Model file for the job. Use its own axes, mm. A direction names the side the tool comes from. Round coordinates to 2 decimals unless told otherwise and drop trailing zeros. Order: outer loops, then holes, each group sorted by start corner. A loop starts at its lowest first (then second) coordinate and runs counter-clockwise, first axis right, second up. Notation, with made-up numbers: (26.25, 17) - (35.25, 17) arc R16 ccw to (35.25, 39) - close; hole circle Ø2 at (28, 34.5). An arc over 180 degrees is marked (long way). Write item = value, one per line.
```python
from build123d import *

# Parameters (mm, degrees)
F0_R     = 127
F1_DEPTH = 25.4
F3_DEPTH = 28.575
F5_DEPTH = 28.575


with BuildPart() as f1:
    # F0 (on Top) → F1 (new body)
    with BuildSketch(Plane.XY):
        Circle(F0_R)
    extrude(amount=F1_DEPTH)

    # F2 (on Right) → F3 (join, symmetric)
    with BuildSketch(Plane.YZ):
        Polygon((-107.95, 42.457951), (-107.95, 25.4), (0, 25.4), (0, 114.3), (-36.107951, 114.3), align=None)
        Polygon((0, 114.3), (0, 25.4), (107.95, 25.4), (107.95, 42.457951), (36.107951, 114.3), align=None)
    extrude(amount=F3_DEPTH, both=True)

    # F4 (on Front) → F5 (join, symmetric)
    with BuildSketch(Plane.XZ):
        Polygon((-114.3, 42.457951), (-114.3, 25.4), (0, 25.4), (0, 114.3), (-42.457951, 114.3), align=None)
        Polygon((0, 114.3), (0, 25.4), (114.3, 25.4), (114.3, 42.457951), (42.457951, 114.3), align=None)
    extrude(amount=F5_DEPTH, both=True)


solid = f1.part
```
1) 3-axis set-ups, long thin cutter, end or side, ignore diameter. For faces 1 (the face through (0, 107.95, 34)), 2 (the face through (0, -107.95, 34)), 3 (the face through (-63, 28.575, 61)), 4 (the face through (-63, -28.575, 61)), 5 (the face through (61, 28.575, 61)): which of +Z, -Z, +X, -X, +Y, -Y reach the whole face in a straight line?
Conclusion:
face_1 = +Z, +X, -X, +Y
face_2 = +Z, +X, -X, -Y
face_3 = +Z, -X, +Y
face_4 = +Z, -X, -Y
face_5 = +Z, +X, +Y
2) Cut at A-A (z = 34). Write the cut outline in (x, y) (3 decimals).
Conclusion:
outline = (-114.3, -28.575) - (-28.575, -28.575) - (-28.575, -107.95) - (28.575, -107.95) - (28.575, -28.575) - (114.3, -28.575) - (114.3, 28.575) - (28.575, 28.575) - (28.575, 107.95) - (-28.575, 107.95) - (-28.575, 28.575) - (-114.3, 28.575) - close
3) Wall check: line 1 along X through (y, z) = (43, 101.5) (3 decimals); line 2 along Z through (x, y) = (-98, -61). Give the ranges that are in metal, low to high.
Conclusion:
line_1 = -28.575 to 28.575
line_2 = 0 to 25.4
4) Cut at D-D (x = 18.5). Write the cut outline in (y, z).
Conclusion:
outline = (-125.65, 0) - (125.65, 0) - (125.65, 25.4) - (107.95, 25.4) - (107.95, 42.46) - (36.11, 114.3) - (-36.11, 114.3) - (-107.95, 42.46) - (-107.95, 25.4) - (-125.65, 25.4) - close
5) Flat gauge pins, fed straight in: pin 1 Ø8.5 at (y, z) = (0, 35) entering from -X; pin 2 Ø8.5 at (y, z) = (10.5, 38) entering from +X; pin 3 Ø5 at (x, z) = (-5, 36) entering from -Y. Where does each tip first touch, or does it go through?
Conclusion:
pin_1 = -114.3
pin_2 = 114.3
pin_3 = -107.95
6) Cut at B-B (y = 0). Write the cut outline in (x, z).
Conclusion:
outline = (-127, 0) - (127, 0) - (127, 25.4) - (114.3, 25.4) - (114.3, 42.46) - (42.46, 114.3) - (-42.46, 114.3) - (-114.3, 42.46) - (-114.3, 25.4) - (-127, 25.4) - close
7) Cut at C-C (x = 47). Write the cut outline in (y, z) (3 decimals).
Conclusion:
outline = (-117.983, 0) - (117.983, 0) - (117.983, 25.4) - (28.575, 25.4) - (28.575, 109.758) - (-28.575, 109.758) - (-28.575, 25.4) - (-117.983, 25.4) - close
